Work out the finished part from the listing and answer in its coordinate system (mm). Give positions to 0.01 mm unless a question says otherwise; leave off trailing zeros. Loops run counter-clockwise (first coordinate to the right, second up) from the corner with the lowest first, then second, coordinate; pieces in that order, holes last. Notation, with made-up numbers: (-31, 45) - (27, 45) arc R14 cw to (27, 62) - close; hole circle Ø10 at (-12, 10). An arc over 180 degrees is marked (long way). One line per question, with ' | ' between items.
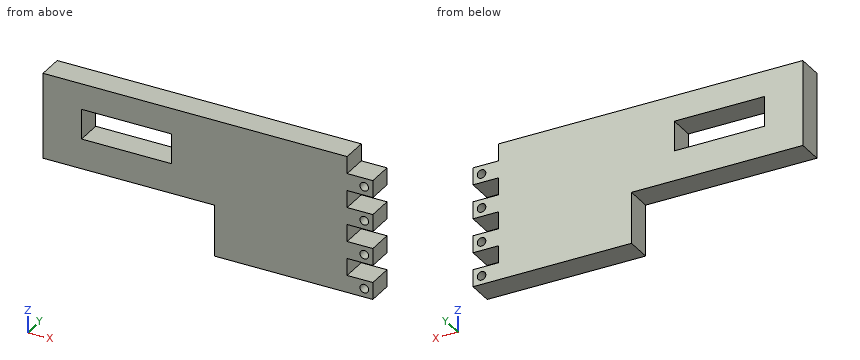
from build123d import *

# Parameters (mm, degrees)
BOSS_EXTRUDE1_DEPTH = 6
SKETCH2_W           = 21
SKETCH2_H           = 7
CUT_EXTRUDE1_DEPTH  = 46.122056691
SKETCH3_R           = 1
CUT_EXTRUDE2_DEPTH  = 46.122056691


with BuildPart() as part:
    # Sketch1 → Boss-Extrude1 (new body)
    with BuildSketch(Plane(origin=(0, 0, 0), x_dir=(1, 0, 0), z_dir=(0, 1, 0))):
        Polygon((-40, 0), (0, 0), (0, 12), (37, 12), (37, 8), (31, 8), (31, 4), (37, 4), (37, 0), (31, 0), (31, -4), (37, -4), (37, -8), (31, -8), (31, -12), (37, -12), (37, -16), (31, -16), (31, -20), (-40, -20), align=None)
    extrude(amount=BOSS_EXTRUDE1_DEPTH)

    # Sketch2 → Cut-Extrude1 (cut, through all)
    with BuildSketch(Plane(origin=(0, 6, 0), x_dir=(1, 0, 0), z_dir=(0, 1, 0))):
        with Locations((-20.5, -10.5)):
            Rectangle(SKETCH2_W, SKETCH2_H)
    extrude(amount=-CUT_EXTRUDE1_DEPTH, mode=Mode.SUBTRACT)

    # Sketch3 → Cut-Extrude2 (cut, through all)
    with BuildSketch(Plane(origin=(0, 6, 0), x_dir=(1, 0, 0), z_dir=(0, 1, 0))):
        with Locations(Location((35, 10, 0), (0, 0, 270))):
            Circle(SKETCH3_R)
        with Locations(Location((35, 2, 0), (0, 0, 270))):
            Circle(SKETCH3_R)
        with Locations(Location((35, -6, 0), (0, 0, 270))):
            Circle(SKETCH3_R)
        with Locations(Location((35, -14, 0), (0, 0, 270))):
            Circle(SKETCH3_R)
    extrude(amount=-CUT_EXTRUDE2_DEPTH, mode=Mode.SUBTRACT)


solid = part.part
1. Flat-ended cylindrical pins translate along their axes: pin 1 (1.2 mm diameter, centred on y = 2.5, z = 9.5, fed in from +X); pin 2 (1.8 mm diameter, centred on x = 33, y = 2.5, fed in from +Z). Find the tip coordinate at first contact, or state that the pin passes through.
Evaluation:
pin 1: x = 31 | pin 2: z = 16
2. Consider L1, parallel to X at y = 4.7, z = 11.5; L2, parallel to Z at x = -28.5, y = 3.55; L3, parallel to X at y = 3.1, z = 6. Determine where each line is inside the solid, lowest interval first.
Evaluation:
L1: -40 to -31, -10 to 31 | L2: 0 to 7, 14 to 20 | L3: -40 to 34, 36 to 37
3. Find section A-A on x = -15. Write down the section's boundary in (y, z), then the cut area to 3 significant figures.
Evaluation:
outline: (0, 0) - (6, 0) - (6, 7) - (0, 7) - close; (0, 14) - (6, 14) - (6, 20) - (0, 20) - close | area: 78.0 mm2
4. Find section C-C on y = 4.55. Write down the section's boundary in (x, z).
Evaluation:
outline: (-40, 0) - (0, 0) - (0, -12) - (37, -12) - (37, -8) - (31, -8) - (31, -4) - (37, -4) - (37, 0) - (31, 0) - (31, 4) - (37, 4) - (37, 8) - (31, 8) - (31, 12) - (37, 12) - (37, 16) - (31, 16) - (31, 20) - (-40, 20) - close; hole (-31, 7) - (-10, 7) - (-10, 14) - (-31, 14) - close; hole circle Ø2 at (35, -10); hole circle Ø2 at (35, -2); hole circle Ø2 at (35, 6); hole circle Ø2 at (35, 14)
5. Find section D-D on x = 35. State how many separate pieces and enclosed holes the cut face has, then the cut area to 3 significant figures.
Evaluation:
separate pieces: 8 | enclosed holes: 0 | area: 48.0 mm2
6. Find section B-B on z = -10. Write down the section's boundary in (x, y), then the cut area to 3 significant figures.
Evaluation:
outline: (0, 0) - (34, 0) - (34, 6) - (0, 6) - close; (36, 0) - (37, 0) - (37, 6) - (36, 6) - close | area: 210 mm2
